Can you work these out from the model? Positions are in its coordinate system, mm. Give positions to 0.01 mm unless a question says otherwise; leave off trailing zeros. Loops run counter-clockwise (first coordinate to the right, second up) from the corner with the lowest first, then second, coordinate; pieces in that order, holes last. Notation, with made-up numbers: (-15, 54) - (23, 54) arc R28 ccw to (23, 72) - close; hole circle Ø3 at (-3, 38). An arc over 180 degrees is marked (long way). Answer as a JSON object with one key per item and string values. Group by question number.
Item 1: Suppose I cut it at A-A on z = 53. Write out the boundary of the cut face in (x, y).
Item 2: Please list where these lines run through material, in increasing order: L1, parallel to X at y = -34.5, z = 53; L2, parallel to X at y = -29.5, z = 51; L3, parallel to Z at x = -1299, y = -35.
Item 3: Suppose I cut it at B-B on x = -1441.5. Write out the boundary of the cut face in (y, z).
Item 4: Will these pins go through, and if not, where does the flat tip stop? pin 1 (1 mm diameter, centred on x = -2203, z = 20.5, fed in from +Y); pin 2 (2 mm diameter, centred on x = -1218.5, z = 29.5, fed in from -Y); pin 3 (6 mm diameter, centred on x = -993.5, y = -20.5, fed in from -Z).
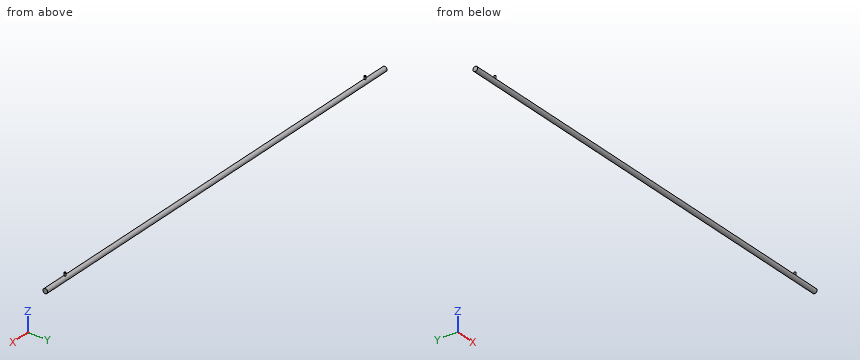
Solid Edge part; units mm, degrees
sketch "Sketch1" plane through (0, 0, 0) normal (1, 0, 0) x (0, 1, 0)
  circle A0 centre (-32.3272, 26.5857) radius 15
extrude "Protrusion1" add sketch "Sketch1" against normal blind 1410
revolve "RevolvedProtrusion1" [suppressed]
sketch "Sketch2" plane through (0, 0, 26.5855) normal (0, 0, 1) x (1, 0, 0)
  circle A0 centre (-163.2288, -32.3267) radius 5
extrude "ExtrudedProtrusion_5" add sketch "Sketch2" along normal blind 35
mirror "Mirror1" about plane through (-1410, -32.3272, 26.5857) normal (-1, 0, 0) of "Protrusion1", "ExtrudedProtrusion_5"
Worked out:
{
 "1": {"outline": "circle Ø10 at (-2656.77, -32.33); circle Ø10 at (-163.23, -32.33)"},
 "2": {"L1": "x = -2661.27 to -2652.27, -167.73 to -158.73", "L2": "x = -2660.9 to -2652.65, -167.35 to -159.1", "L3": "z = 11.83 to 41.35"},
 "3": {"outline": "circle Ø30 at (-32.33, 26.59)"},
 "4": {"pin 1": "stops at y = -18.41", "pin 2": "stops at y = -47.2", "pin 3": "stops at z = 14.46"}
}
